```python
from build123d import *

# Parameters (mm, degrees)
ESBO_O1_W                = 20
ESBO_O1_H                = 40
ESBO_O1_R                = 8
RESSALTO_EXTRUS_O1_DEPTH = 2.5
ESBO_O2_R                = 2.6
CORTE_EXTRUS_O1_DEPTH    = 23.912878475
FILETE1_R                = 5


with BuildPart() as part:
    # Esboço1 → Ressalto-extrusão1 (new, symmetric)
    with BuildSketch(Plane.XY):
        Rectangle(ESBO_O1_W, ESBO_O1_H)
        Circle(ESBO_O1_R, mode=Mode.SUBTRACT)
    extrude(amount=RESSALTO_EXTRUS_O1_DEPTH, both=True)

    # Esboço2 → Corte-extrusão1 (cut, through all)
    with BuildSketch(Plane.XY.offset(2.5)):
        with Locations((0, -15)):
            Circle(ESBO_O2_R)
    corte_extrus_o1 = extrude(amount=-CORTE_EXTRUS_O1_DEPTH, mode=Mode.SUBTRACT)

    # Espelhar1: Corte-extrusão1 across plane
    add(corte_extrus_o1.mirror(Plane.ZX), mode=Mode.SUBTRACT)

    # Filete1
    filete1_edges = [part.edges().sort_by_distance(p)[0] for p in [
        (10, -20, 0),
        (-10, -20, 0),
        (-10, 20, 0),
        (10, 20, 0),
    ]]
    fillet(filete1_edges, radius=FILETE1_R)


solid = part.part
```
Could you check a few things on this model? Use its own coordinates, in mm. Round coordinates to 2 decimals unless told otherwise and drop trailing zeros. Write each loop counter-clockwise with the first axis right and the second up, starting at its lowest first coordinate (ties: lowest second). Pieces come first, ordered by that corner, then holes. Notation, with made-up numbers: M -30,37.5 L 6,37.5 A12 cw 6,57.5 Z; hole C 14.5,61.5 d9. An arc over 180 degrees is marked long. Answer in a Markdown table with one row per item. Add a question column.
Q1. If I drill on line 1 (Y direction, x = 0, z = -1.2); line 2 (Y direction, x = 1.25, z = 0.9); line 3 (X direction, y = 15, z = 0.7), over which ranges is the centre line in solid material (lowest first)? Write a range as from..to.
Q2. If we mould it in two halves opening along Y, with no side actions, what happens to faces 1 (the cylindrical face through (-9, -18, 0)), 2 (the flat face through (7, 5, -2.5)), 3 (the cylindrical face through (-1.73, -7.81, -0.04))? For each: +Y half, -Y half, draft (parallel to the pull), parting line (faces both ways), or undercut.
Q3. Imagine slicing it at C-C (z = -0.25). Please give me the cut outline in (x, y).
Q4. Will these pins go through, and if not, where does the flat tip stop? pin 1 Ø1 at (y, z) = (15.5, 1) entering from +X; pin 2 Ø3 at (x, y) = (0, 15) entering from -Z.
Q5. Imagine slicing it at A-A (x = 0). Please give me the cut outline in (y, z).
Q6. Imagine slicing it at D-D (x = 6.75). Please give me the cut outline in (y, z), then the cut area to 3 significant figures.
Q7. Imagine slicing it at B-B (y = -14). Please give me the cut outline in (x, z), then the cut area to 3 significant figures.
Values:
| question | item | result |
|---|---|---|
| 1 | line 1 | -20..-17.6, -12.4..-8, 8..12.4, 17.6..20 |
| 1 | line 2 | -20..-17.28, -12.72..-7.9, 7.9..12.72, 17.28..20 |
| 1 | line 3 | -10..-2.6, 2.6..10 |
| 2 | face 1 | -Y half |
| 2 | face 2 | draft |
| 2 | face 3 | undercut |
| 3 | outline | M -10,-15 A5 ccw -5,-20 L 5,-20 A5 ccw 10,-15 L 10,15 A5 ccw 5,20 L -5,20 A5 ccw -10,15 Z; hole C 0,0 d16; hole C 0,-15 d5.2; hole C 0,15 d5.2 |
| 4 | pin 1 | x = 10 |
| 4 | pin 2 | through |
| 5 | outline | M -20,-2.5 L -17.6,-2.5 L -17.6,2.5 L -20,2.5 Z; M -12.4,-2.5 L -8,-2.5 L -8,2.5 L -12.4,2.5 Z; M 8,-2.5 L 12.4,-2.5 L 12.4,2.5 L 8,2.5 Z; M 17.6,-2.5 L 20,-2.5 L 20,2.5 L 17.6,2.5 Z |
| 6 | outline | M -19.68,-2.5 L -4.29,-2.5 L -4.29,2.5 L -19.68,2.5 Z; M 4.29,-2.5 L 19.68,-2.5 L 19.68,2.5 L 4.29,2.5 Z |
| 6 | area | 154 mm^2 |
| 7 | outline | M -10,-2.5 L -2.4,-2.5 L -2.4,2.5 L -10,2.5 Z; M 2.4,-2.5 L 10,-2.5 L 10,2.5 L 2.4,2.5 Z |
| 7 | area | 76.0 mm^2 |
